Check sheet for the modelled part. Datum: model origin and axes. Units: mm. A direction names the side the tool comes from. Give positions to 0.01 mm unless a question says otherwise; leave off trailing zeros. Order: outer loops, then holes, each group sorted by start corner. A loop starts at its lowest first (then second) coordinate and runs counter-clockwise, first axis right, second up. Notation, with made-up numbers: M 61.5,37 L 98.5,37 A31 ccw 98.5,73 Z; hole C -32.75,-0.5 d7. An arc over 180 degrees is marked long. One line per question, with ' | ' between items. Start each with the question number.
```python
from build123d import *

# Parameters (mm, degrees)
SKETCH_1_W          = 24.2
SKETCH_1_H          = 42.3
EXTRUDE_1_DEPTH     = 6.7
FILLET_1_R          = 4
CUT_EXTRUDE_1_DEPTH = 5.7
CUT_EXTRUDE_2_DEPTH = 26.024438056
CHAMFER_1_SIZE      = 0.5
CHAMFER_2_SIZE      = 1
CUT_EXTRUDE_3_DEPTH = 3.6
EXTRUDE_START       = 3.6
EXTRUDE_2_DEPTH     = 3.6
CUT_EXTRUDE_5_DEPTH = 2.1
FILLET_4_R          = 2.5
M2X0_4_3_D          = 1.6
M2X0_4_3_DEPTH      = 5.019311505
M2X0_4_3_TIP        = 0.480688495
SKETCH_14_W         = 7.5
SKETCH_14_H         = 1
CUT_EXTRUDE_6_DEPTH = 3.6
SKETCH_15_W         = 9.4
SKETCH_15_H         = 1.594635817
CUT_EXTRUDE_7_DEPTH = 3.6


with BuildPart() as part:
    # 草图1 → 凸台-拉伸1 (new body)
    with BuildSketch(Plane(origin=(0, 0, 0), x_dir=(1, 0, 0), z_dir=(0, 1, 0))):
        Rectangle(SKETCH_1_W, SKETCH_1_H)
    extrude(amount=EXTRUDE_1_DEPTH)

    # 圆角1
    fillet_1_edges = [part.edges().sort_by_distance(p)[0] for p in [
        (12.1, 3.35, 21.15),
        (-12.1, 3.35, 21.15),
        (-12.1, 3.35, -21.15),
        (12.1, 3.35, -21.15),
    ]]
    fillet(fillet_1_edges, radius=FILLET_1_R)

    # 草图2 → 切除-拉伸1 (cut)
    with BuildSketch(Plane.XZ):
        with BuildLine():
            Line((-6.3, -18.15), (6.3, -18.15))
            ThreePointArc((6.3, -18.15), (8.279898987, -17.329898987), (9.1, -15.35))
            Line((9.1, -15.35), (9.1, 15.35))
            ThreePointArc((9.1, 15.35), (8.279898987, 17.329898987), (6.3, 18.15))
            Line((6.3, 18.15), (-6.3, 18.15))
            ThreePointArc((-6.3, 18.15), (-8.279898987, 17.329898987), (-9.1, 15.35))
            Line((-9.1, 15.35), (-9.1, -15.35))
            ThreePointArc((-9.1, -15.35), (-8.279898987, -17.329898987), (-6.3, -18.15))
        make_face()
    extrude(amount=-CUT_EXTRUDE_1_DEPTH, mode=Mode.SUBTRACT)

    # 草图3 → 切除-拉伸2 (cut, through all)
    with BuildSketch(Plane.XZ.offset(-5.7)):
        with BuildLine():
            Line((-6.3, -17.15), (6.3, -17.15))
            ThreePointArc((6.3, -17.15), (7.572792206, -16.622792206), (8.1, -15.35))
            Line((8.1, -15.35), (8.1, 13.45))
            ThreePointArc((8.1, 13.45), (7.572792206, 14.722792206), (6.3, 15.25))
            Line((6.3, 15.25), (-6.3, 15.25))
            ThreePointArc((-6.3, 15.25), (-7.572792206, 14.722792206), (-8.1, 13.45))
            Line((-8.1, 13.45), (-8.1, -15.35))
            ThreePointArc((-8.1, -15.35), (-7.572792206, -16.622792206), (-6.3, -17.15))
        make_face()
    extrude(amount=-CUT_EXTRUDE_2_DEPTH, mode=Mode.SUBTRACT)

    # 倒角1
    chamfer_1_edges = [part.edges().sort_by_distance(p)[0] for p in [
        (-7.572792206, 6.7, 14.722792206),
        (0, 6.7, 15.25),
        (7.572792206, 6.7, 14.722792206),
        (8.1, 6.7, -0.95),
        (7.572792206, 6.7, -16.622792206),
        (0, 6.7, -17.15),
        (-7.572792206, 6.7, -16.622792206),
        (-8.1, 6.7, -0.95),
    ]]
    chamfer(chamfer_1_edges, length=CHAMFER_1_SIZE)

    # 倒角2
    chamfer_2_edges = [part.edges().sort_by_distance(p)[0] for p in [
        (12.1, 6.7, 0),
        (0, 6.7, 21.15),
        (0, 6.7, -21.15),
        (-12.1, 6.7, 0),
        (-10.928427125, 6.7, 19.978427125),
        (10.928427125, 6.7, -19.978427125),
        (-10.928427125, 6.7, -19.978427125),
        (10.928427125, 6.7, 19.978427125),
    ]]
    chamfer(chamfer_2_edges, length=CHAMFER_2_SIZE)

    # 草图4 → 切除-拉伸3 (cut)
    with BuildSketch(Plane.XZ):
        with BuildLine():
            Line((11.1, -17.15), (11.1, 17.15))
            ThreePointArc((11.1, 17.15), (10.221320344, 19.271320344), (8.1, 20.15))
            Line((8.1, 20.15), (-8.1, 20.15))
            ThreePointArc((-8.1, 20.15), (-10.221320344, 19.271320344), (-11.1, 17.15))
            Line((-11.1, 17.15), (-11.1, -17.15))
            ThreePointArc((-11.1, -17.15), (-10.221320344, -19.271320344), (-8.1, -20.15))
            Line((-8.1, -20.15), (8.1, -20.15))
            ThreePointArc((8.1, -20.15), (10.221320344, -19.271320344), (11.1, -17.15))
        make_face()
    extrude(amount=-CUT_EXTRUDE_3_DEPTH, mode=Mode.SUBTRACT)

    # 草图7 → 凸台-拉伸2 (add)
    with BuildSketch(Plane.XZ.offset(-3.6).offset(EXTRUDE_START)):
        with BuildLine():
            Line((6.758096095, 20.15), (8.1, 20.15))
            ThreePointArc((8.1, 20.15), (10.221320344, 19.271320344), (11.1, 17.15))
            Line((11.1, 17.15), (11.1, 15.808096095))
            Line((11.1, 15.808096095), (9.062272247, 15.808096095))
            ThreePointArc((9.062272247, 15.808096095), (8.279898987, 17.329898987), (6.758096095, 18.112272247))
            Line((6.758096095, 18.112272247), (6.758096095, 20.15))
        make_face()
        with BuildLine():
            Line((-6.758096095, 20.15), (-8.1, 20.15))
            ThreePointArc((-8.1, 20.15), (-10.221320344, 19.271320344), (-11.1, 17.15))
            Line((-11.1, 17.15), (-11.1, 15.808096095))
            Line((-11.1, 15.808096095), (-9.062272247, 15.808096095))
            ThreePointArc((-9.062272247, 15.808096095), (-8.279898987, 17.329898987), (-6.758096095, 18.112272247))
            Line((-6.758096095, 18.112272247), (-6.758096095, 20.15))
        make_face()
        with BuildLine():
            Line((-8.1, -20.15), (-6.758096095, -20.15))
            Line((-6.758096095, -20.15), (-6.758096095, -18.112272247))
            ThreePointArc((-6.758096095, -18.112272247), (-8.279898987, -17.329898987), (-9.062272247, -15.808096095))
            Line((-9.062272247, -15.808096095), (-11.1, -15.808096095))
            Line((-11.1, -15.808096095), (-11.1, -17.15))
            ThreePointArc((-11.1, -17.15), (-10.221320344, -19.271320344), (-8.1, -20.15))
        make_face()
        with BuildLine():
            Line((11.1, -17.15), (11.1, -15.808096095))
            Line((11.1, -15.808096095), (9.062272247, -15.808096095))
            ThreePointArc((9.062272247, -15.808096095), (8.279898987, -17.329898987), (6.758096095, -18.112272247))
            Line((6.758096095, -18.112272247), (6.758096095, -20.15))
            Line((6.758096095, -20.15), (8.1, -20.15))
            ThreePointArc((8.1, -20.15), (10.221320344, -19.271320344), (11.1, -17.15))
        make_face()
    extrude(amount=-EXTRUDE_2_DEPTH)

    # 草图13 → 切除-拉伸5 (cut)
    with BuildSketch(Plane.XZ.offset(-3.6)):
        with BuildLine():
            Line((6.758096095, 18.112272247), (6.758096095, 20.15))
            Line((6.758096095, 20.15), (-6.758096095, 20.15))
            Line((-6.758096095, 20.15), (-6.758096095, 18.112272247))
            ThreePointArc((-6.758096095, 18.112272247), (-6.529823528, 18.140552122), (-6.3, 18.15))
            Line((-6.3, 18.15), (6.3, 18.15))
            ThreePointArc((6.3, 18.15), (6.529823528, 18.140552122), (6.758096095, 18.112272247))
        make_face()
    extrude(amount=-CUT_EXTRUDE_5_DEPTH, mode=Mode.SUBTRACT)

    # 圆角4
    # the kernel refuses this fillet: 2.5 mm, written as the material it adds along each edge
    with BuildSketch(Plane(origin=(-11.1, 0, 15.808096095), x_dir=(0, 0, -1), z_dir=(0, 1, 0)), Plane(origin=(11.1, 0, -15.808096095), x_dir=(0, 0, 1), z_dir=(0, 1, 0)), Plane(origin=(-6.758096095, 0, -20.15), x_dir=(1, 0, 0), z_dir=(0, 1, 0))) as fillet_4_piece_1:
        with BuildLine():
            CenterArc((2.456889165, -2.5), FILLET_4_R, 90, 79.34417895)
            Line((0, -2.037727753), (-0.049137783, -2.028482308))
            ThreePointArc((-0.049137783, -2.028482308), (-0.05, -1.018863876), (-0.05, 0))
            Line((-0.05, 0), (0, 0.05))
            Line((0, 0.05), (2.456889165, 0.05))
            Line((2.456889165, 0.05), (2.456889165, 0))
        make_face()
    extrude(amount=3.6)
    with BuildSketch(Plane(origin=(-6.758096095, 0, 20.15), x_dir=(0, 0, -1), z_dir=(0, 1, 0))) as fillet_4_piece_2:
        with BuildLine():
            CenterArc((2.5, -2.456889165), FILLET_4_R, 100.65582105, 79.34417895)
            Line((0, -2.456889165), (-0.05, -2.456889165))
            Line((-0.05, -2.456889165), (-0.05, 0))
            Line((-0.05, 0), (0, 0.05))
            ThreePointArc((0, 0.05), (1.018863876, 0.05), (2.028482308, 0.049137783))
            Line((2.028482308, 0.049137783), (2.037727753, 0))
        make_face()
    extrude(amount=5.7)
    with BuildSketch(Plane(origin=(6.758096095, 0, 20.15), x_dir=(-1, 0, 0), z_dir=(0, 1, 0))) as fillet_4_piece_3:
        with BuildLine():
            CenterArc((2.456889165, -2.5), FILLET_4_R, 90, 79.34417895)
            Line((0, -2.037727753), (-0.049137783, -2.028482308))
            ThreePointArc((-0.049137783, -2.028482308), (-0.05, -1.018863876), (-0.05, 0))
            Line((-0.05, 0), (0, 0.05))
            Line((0, 0.05), (2.456889165, 0.05))
            Line((2.456889165, 0.05), (2.456889165, 0))
        make_face()
    extrude(amount=5.7)
    with BuildSketch(Plane(origin=(11.1, 0, 15.808096095), x_dir=(-1, 0, 0), z_dir=(0, 1, 0)), Plane(origin=(-11.1, 0, -15.808096095), x_dir=(1, 0, 0), z_dir=(0, 1, 0)), Plane(origin=(6.758096095, 0, -20.15), x_dir=(0, 0, 1), z_dir=(0, 1, 0))) as fillet_4_piece_4:
        with BuildLine():
            CenterArc((2.5, -2.456889165), FILLET_4_R, 100.65582105, 79.34417895)
            Line((0, -2.456889165), (-0.05, -2.456889165))
            Line((-0.05, -2.456889165), (-0.05, 0))
            Line((-0.05, 0), (0, 0.05))
            ThreePointArc((0, 0.05), (1.018863876, 0.05), (2.028482308, 0.049137783))
            Line((2.028482308, 0.049137783), (2.037727753, 0))
        make_face()
    extrude(amount=3.6)

    # M2x0.4 螺纹孔3
    with Locations(Plane(origin=(0, 0, 0), x_dir=(-1, 0, 0), z_dir=(0, -1, 0))):
        with Locations((-9.6, 18.65), (9.6, 18.65), (9.6, -18.65), (-9.6, -18.65)):
            Hole(M2X0_4_3_D / 2, depth=M2X0_4_3_DEPTH)
            with Locations((0, 0, -(M2X0_4_3_DEPTH + M2X0_4_3_TIP / 2))):  # 118° drill point
                Cone(0, M2X0_4_3_D / 2, M2X0_4_3_TIP, mode=Mode.SUBTRACT)

    # 草图14 → 切除-拉伸6 (cut)
    with BuildSketch(Plane.XZ):
        with Locations((0, -20.65)):
            Rectangle(SKETCH_14_W, SKETCH_14_H)
    extrude(amount=-CUT_EXTRUDE_6_DEPTH, mode=Mode.SUBTRACT)

    # 草图15 → 切除-拉伸7 (cut)
    with BuildSketch(Plane.XZ):
        with Locations((0, 20.352682092)):
            Rectangle(SKETCH_15_W, SKETCH_15_H)
    extrude(amount=-CUT_EXTRUDE_7_DEPTH, mode=Mode.SUBTRACT)


solid = part.part
```
Item 1: Scan lines: probe 1 along Z at (x, y) = (-9.6, 3.1); probe 2 along X at (y, z) = (1.5, -5); probe 3 along Z at (x, y) = (-10.25, 5). Record each from-to range of solid material in increasing order. Write a range as [from, to].
Item 2: Set-up check for faces 5 (the face through (7.587, 5.946, 14.709)), 6 (the face through (-5.88, 1.77, -19.59)), 7 (the face through (-7.653, 6.335, 14.833)), 8 (the face through (3.75, 1.8, -20.7)): record each of +Z, -Z, +X, -X, +Y, -Y from which the full face is reachable in a straight line by a thin tool's end or side.
Item 3: Section check D-D, the plane x = 5.75. Record the cut outline in (y, z).
Item 4: Section check A-A, the plane z = -4. Record the cut outline in (x, y), then the cut area to 4 significant figures.
Item 5: Section check C-C, the plane x = 1.25. Record the cut outline in (y, z).
Item 6: Section check B-B, the plane y = 1. State how many separate pieces and enclosed holes the cut face has, then the cut area to 3 significant figures.
Item 7: Draft check along X on faces 1 (the face through (-10.448, 6.415, 19.447)), 2 (the face through (-9.1, 5, 0)), 3 (the face through (-0.11, 6.19, 20.66)), 4 (the face through (5.916, 1.775, -19.559)). Enter one of: released by +X, released by -X, zero draft, split by the parting line, or undercut.
Item 8: Go/stop test with flat-tipped pins: P1, Ø1.3, axis at x = -9.6, z = -18.65, coming from the -Y side; P2, Ø2.5, axis at x = -0.5, z = -20, coming from the -Y side; P3, Ø10, axis at x = 3, z = -10.5, coming from the +Y side. Record where each tip stops, or that it passes through.
Reported:
1) probe 1: z = [-20.86, -19.45], [-17.85, -15.64], [15.64, 17.85], [19.45, 20.86] | probe 2: x = [-12.1, -11.1], [11.1, 12.1] | probe 3: z = [-20.52, -19.12], [-18.18, 18.18], [19.12, 20.52]
2) face 5: +Y, -Y | face 6: -Y | face 7: +Y | face 8: +Z, -Z, -Y
3) outline: M 0,-21.15 L 5.7,-21.15 L 6.7,-20.15 L 6.7,-17.65 L 6.2,-17.15 L 5.7,-17.15 L 5.7,-18.15 L 3.6,-18.15 L 3.6,-19.69 L 0,-19.69 Z; M 0,19.69 L 5.7,19.69 L 5.7,15.25 L 6.2,15.25 L 6.7,15.75 L 6.7,20.15 L 5.7,21.15 L 0,21.15 Z
4) outline: M -12.1,0 L -11.1,0 L -11.1,3.6 L -9.1,3.6 L -9.1,5.7 L -8.1,5.7 L -8.1,6.2 L -8.6,6.7 L -11.1,6.7 L -12.1,5.7 Z; M 8.1,5.7 L 9.1,5.7 L 9.1,3.6 L 11.1,3.6 L 11.1,0 L 12.1,0 L 12.1,5.7 L 11.1,6.7 L 8.6,6.7 L 8.1,6.2 Z | area: 26.55 mm^2
5) outline: M 3.6,-21.15 L 5.7,-21.15 L 6.7,-20.15 L 6.7,-17.65 L 6.2,-17.15 L 5.7,-17.15 L 5.7,-18.15 L 3.6,-18.15 Z; M 3.6,20.15 L 5.7,20.15 L 5.7,15.25 L 6.2,15.25 L 6.7,15.75 L 6.7,20.15 L 5.7,21.15 L 3.6,21.15 Z
6) separate pieces: 2 | enclosed holes: 4 | area: 160 mm^2
7) face 1: released by -X | face 2: undercut | face 3: zero draft | face 4: undercut
8) P1: stops at y = 5.11 | P2: stops at y = 3.6 | P3: passes through
